Input: dimensioned drawing with shaded views. Units: mm. Origin: part minimum x, y, z. Coordinates: 2 decimals unless noted, no trailing zeros. Loops run counter-clockwise (first coordinate to the right, second up) from the corner with the lowest first, then second, coordinate; pieces in that order, holes last. Notation, with made-up numbers: M 69.5,47.25 L 91.5,47.25 A18 ccw 91.5,73.25 Z; hole C 85.25,26 d6. An arc over 180 degrees is marked long. Write item = value, one per line. Start each with the question number.
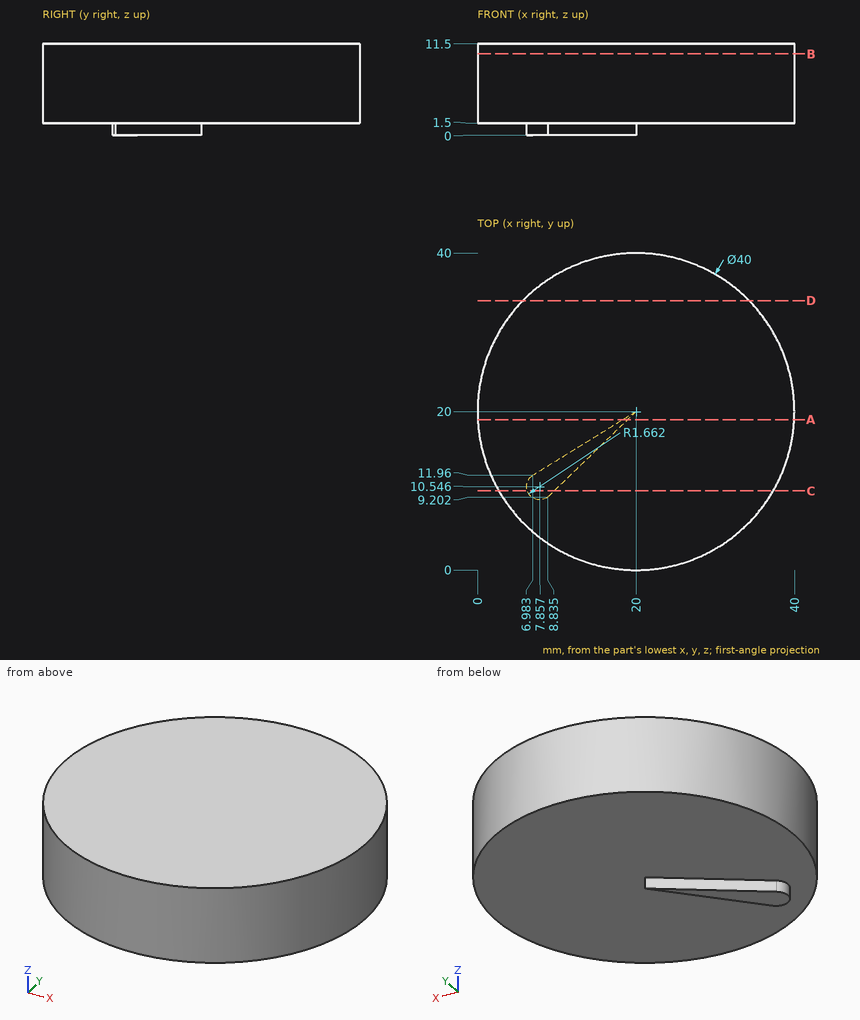
Item 1: Section query C-C (y = 10). Return the cut outline in (x, z).
Item 2: Section query D-D (y = 34). Return the cut outline in (x, z), plus the area to 3 significant figures.
Item 3: First-contact query: pin 1 (10 mm diameter, centred on x = 33.5, y = 13, fed in from -Z); pin 2 (2 mm diameter, centred on y = 4, z = 4.5, fed in from -X). Flat tips, straight axial feed; report the tip coordinate or a pass-through.
Item 4: Line query: line 1 (Z direction, x = 36, y = 17); line 2 (X direction, y = 38.5, z = 5.5) (1 decimal); line 3 (Y direction, x = 10.5, z = 1.25). Output: solid intervals per line, ascending. Write a range as from..to.
Item 5: Section query B-B (z = 10.25). Return the cut outline in (x, y).
Item 6: Section query A-A (y = 19). Return the cut outline in (x, z) (1 decimal).
Verdict:
q1.outline = M 2.68,1.5 L 6.29,1.5 L 6.29,0 L 9.66,0 L 9.66,1.5 L 37.32,1.5 L 37.32,11.5 L 2.68,11.5 Z
q2.outline = M 5.72,1.5 L 34.28,1.5 L 34.28,11.5 L 5.72,11.5 Z
q2.area = 286 mm2
q3.pin_1 = 1.5
q3.pin_2 = 6.77
q4.line_1 = 1.5..11.5
q4.line_2 = 12.4..27.6
q4.line_3 = 10.81..14.13
q5.outline = C 20,20 d40
q6.outline = M 0,1.5 L 18.4,1.5 L 18.4,0 L 19,0 L 19,1.5 L 40,1.5 L 40,11.5 L 0,11.5 Z
